Check sheet for the modelled part. Datum: model origin and axes. Units: mm. A direction names the side the tool comes from. Round coordinates to 2 decimals unless told otherwise and drop trailing zeros. Order: outer loops, then holes, each group sorted by start corner. A loop starts at its lowest first (then second) coordinate and runs counter-clockwise, first axis right, second up. Notation, with made-up numbers: (5, 33.25) -> (57, 33.25) arc R13 ccw to (57, 51.25) -> close; hole circle Ø9 at (86.25, -35.75). An arc over 180 degrees is marked (long way). Answer in a Markdown table with one row per item.
Autodesk Inventor part; units mm, degrees
ref_plane "YZ Plane" through (0, 0, 0) normal (1, 0, 0) x (0, 1, 0)
ref_plane "XZ Plane" through (0, 0, 0) normal (0, 1, 0) x (-1, 0, 0)
ref_plane "XY Plane" through (0, 0, 0) normal (0, 0, 1) x (1, 0, 0)
sketch "Sketch1" plane through (0, 0, 0) normal (1, 0, 0) x (0, 1, 0)
  line L0 (0, 0) -> (0, 22)
  line L1 (0, 22) -> (2, 22)
  line L2 (2, 22) -> (2, 20)
  line L3 (2, 20) -> (72, 20)
  line L4 (72, 20) -> (72, 22)
  line L5 (72, 22) -> (74, 22)
  line L6 (74, 22) -> (74, 0)
  line L7 (74, 0) -> (0, 0)
  point P0 (74, 11)
  dimension "d0" = 22
  dimension "d5" = 70
  dimension "d6" = 2
  dimension "d7" = 2
  dimension "d29" = 2
revolve "Revolution1" add sketch "Sketch1" angle 360 about axis through (0, 74, 0) along (0, -1, 0)
chamfer "Chamfer1" distance 2 angle 45 2 edges at (0, 2, -20) (0, 72, -20)
sketch "Sketch2" plane through (0, 74, 0) normal (0, 1, 0) x (1, 0, 0)
  circle A0 centre (0, 0) radius 22
  circle A1 centre (0, 0) radius 11.05
  dimension "d12" = 22.1
extrude "Extrusion1" cut sketch "Sketch2" against normal blind 56 contours A1
sketch "Sketch3" plane through (0, 0, 0) normal (0, -1, 0) x (1, 0, 0)
  circle A0 centre (0, 0) radius 22
  circle A1 centre (0, 0) radius 11.05
extrude "Extrusion2" cut sketch "Sketch3" against normal blind 7 contours A1
sketch "Sketch4" plane through (0, 7, 0) normal (0, -1, 0) x (1, 0, 0)
  circle A0 centre (0, 0) radius 11.05
  circle A1 centre (0, 0) radius 7.55
  dimension "d18" = 15.1
extrude "Extrusion3" cut sketch "Sketch4" against normal through all contours A1
chamfer "Chamfer2" distance 3.5 angle 45 1 edges at (-7.55, 7, 0)
sketch "Sketch5" plane through (0, 74, 0) normal (0, 1, 0) x (1, 0, 0)
  circle A0 centre (0, 0) radius 11.05
  circle A1 centre (0, 0) radius 20
  circle A2 centre (0, 0) radius 18
  dimension "d25" = 8.95
  dimension "d26" = 2
extrude "Extrusion4" cut sketch "Sketch5" against normal blind 49 contours A2
properties part number "spool holder"
(1) Section check C-C on y = 37.5. Record the boundary of the cut face in (x, z), plus the area to 3 significant figures.
Solutions:
| item | result |
|---|---|
| outline | circle Ø40 at (0, 0); hole circle Ø36 at (0, 0) |
| area | 239 mm^2 |
(2) Tool access check on faces 1 (the cylindrical face through (-2.343, 49.843, -17.847)), 2 (the conical face through (-19.65, 70.13, -4.36)), 3 (the cylindrical face through (-2.395, 3.451, -10.787)). Record the directions out of +Z, -Z, +X, -X, +Y, -Y that give a thin tool (end or side, any length) a straight path to the whole face; none if there is none.
Solutions:
| item | result |
|---|---|
| face 1 | +Y |
| face 2 | none |
| face 3 | -Y |
(3) Depth check by flat-ended pin: pin 1 Ø11 at (x, z) = (6.5, 1.5) entering from +Y; pin 2 Ø17.5 at (x, z) = (0, 0) entering from -Y; pin 3 Ø21.5 at (x, z) = (0, 0) entering from -Y. Enter the tip coordinate at first touch or a pass-through.
Solutions:
| item | result |
|---|---|
| pin 1 | y = 25 |
| pin 2 | y = 9.3 |
| pin 3 | y = 7.3 |
(4) Scan lines: probe 1 along Z at (x, y) = (0, 14); probe 2 along X at (y, z) = (39, 0); probe 3 along Y at (x, z) = (-11.5, 9). Record each from-to range of solid material in increasing order. Write a range as from..to.
Solutions:
| item | result |
|---|---|
| probe 1 | -20..-7.55, 7.55..20 |
| probe 2 | -20..-18, 18..20 |
| probe 3 | 0..25 |
(5) Draft check along X on faces 4 (the flat face through (-10.1, 0, -5.2)), 5 (the flat face through (5, 18, 7)), 6 (the conical face through (19.65, 3.87, -4.36)). Enter one of: pulls with the +X half, pulls with the -X half, needs draft (parallel to the pull), parting line crosses it, or undercut.
Solutions:
| item | result |
|---|---|
| face 4 | needs draft |
| face 5 | undercut |
| face 6 | parting line crosses it |
(6) Section check D-D on y = 21. Record the boundary of the cut face in (x, z).
Solutions:
| item | result |
|---|---|
| outline | circle Ø40 at (0, 0); hole circle Ø22.1 at (0, 0) |
